The listing builds one solid part. Answer for the finished solid, in the listing's coordinates (mm). Round coordinates to 2 decimals unless told otherwise and drop trailing zeros. Order: outer loops, then holes, each group sorted by start corner. A loop starts at its lowest first (then second) coordinate and runs counter-clockwise, first axis right, second up. Notation, with made-up numbers: (88, 89.25) -> (105, 89.25) arc R20 ccw to (105, 112.25) -> close; hole circle Ø10 at (45.5, 84). An arc over 180 degrees is marked (long way). Return JSON: item names as keys, results as strings. Group by question number.
(1) The part is cut by section B-B (z = 5). Determine the outline of the cut face in (x, y), plus the area to 3 significant figures.
(2) Determine the mould class of faces 1 (the face through (0.08, 0, 2.48)), 2 (the face through (-1, -0.25, 1)) for opening direction X: +X half, -X half, draft (parallel to the pull), parting line (faces both ways), or undercut.
(3) Consider line 1 (Z direction, x = 0, y = 0.15) (3 decimals); line 2 (X direction, y = 0.2, z = 5.25); line 3 (Z direction, x = -0.95, y = 0). Determine where each line is inside the solid, lowest interval first. Write a range as [from, to].
(4) The part is cut by section D-D (x = -1.1). Determine the outline of the cut face in (y, z).
(5) The part is cut by section A-A (x = 0). Determine the outline of the cut face in (y, z) (3 decimals).
(6) The part is cut by section C-C (y = -0.1). Determine the outline of the cut face in (x, z) (3 decimals).
from build123d import *

# Parameters (mm, degrees)
SKETCH_R  = 0.65
PAD_DEPTH = 0.25


with BuildPart() as part:
    # Sketch → Pad (new body, symmetric)
    with BuildSketch(Plane(origin=(0, 0, 0), x_dir=(-1, 0, 0), z_dir=(0, 1, 0))):
        with BuildLine():
            Line((-1.25, 5.5), (-1.25, 0))
            Line((-1.25, 0), (-0.6, 0))
            Line((-0.6, 0), (-0.6, -2.4))
            ThreePointArc((-0.6, -2.4), (0, -3), (0.6, -2.4))
            Line((0.6, 0), (0.6, -2.4))
            Line((0.6, 0), (1.25, 0))
            Line((1.25, 0), (1.25, 5.5))
            Line((1.25, 5.5), (0.65, 5.5))
            Line((0.65, 5.5), (0.65, 4.275))
            ThreePointArc((-0.65, 4.275), (0, 3.625), (0.65, 4.275))
            Line((-0.65, 4.275), (-0.65, 5.5))
            Line((-0.65, 5.5), (-1.25, 5.5))
        make_face()
        with Locations((0, 1.83315)):
            Circle(SKETCH_R, mode=Mode.SUBTRACT)
    extrude(amount=PAD_DEPTH, both=True)


solid = part.part
Answer below:
{
 "1": {"outline": "(-1.25, -0.25) -> (-0.65, -0.25) -> (-0.65, 0.25) -> (-1.25, 0.25) -> close; (0.65, -0.25) -> (1.25, -0.25) -> (1.25, 0.25) -> (0.65, 0.25) -> close", "area": "0.600 mm²"},
 "2": {"face 1": "undercut", "face 2": "draft"},
 "3": {"line 1": "z = [-3, 1.183], [2.483, 3.625]", "line 2": "x = [-1.25, -0.65], [0.65, 1.25]", "line 3": "z = [0, 5.5]"},
 "4": {"outline": "(-0.25, 0) -> (0.25, 0) -> (0.25, 5.5) -> (-0.25, 5.5) -> close"},
 "5": {"outline": "(-0.25, -3) -> (0.25, -3) -> (0.25, 1.183) -> (-0.25, 1.183) -> close; (-0.25, 2.483) -> (0.25, 2.483) -> (0.25, 3.625) -> (-0.25, 3.625) -> close"},
 "6": {"outline": "(-1.25, 0) -> (-0.6, 0) -> (-0.6, -2.4) arc R0.6 ccw to (0.6, -2.4) -> (0.6, 0) -> (1.25, 0) -> (1.25, 5.5) -> (0.65, 5.5) -> (0.65, 4.275) arc R0.65 cw to (-0.65, 4.275) -> (-0.65, 5.5) -> (-1.25, 5.5) -> close; hole circle Ø1.3 at (0, 1.833)"}
}
